Autodesk Inventor part; units mm, degrees
ref_plane "YZ Plane" through (0, 0, 0) normal (1, 0, 0) x (0, 1, 0)
ref_plane "XZ Plane" through (0, 0, 0) normal (0, 1, 0) x (-1, 0, 0)
ref_plane "XY Plane" through (0, 0, 0) normal (0, 0, 1) x (1, 0, 0)
sketch "Sketch1" plane through (0, 0, 0) normal (0, 1, 0) x (-1, 0, 0)
  circle A0 centre (368.3, 203.2) radius 2.54 construction
  circle A1 centre (368.3, 241.3) radius 3.302
  circle A2 centre (368.3, 127) radius 2.54 construction
  circle A3 centre (368.3, 88.9) radius 3.302
  circle A4 centre (368.3, 50.8) radius 2.54 construction
  circle A5 centre (368.3, 12.7) radius 3.302
  line L0 (190.5, 244.602) -> (330.2, 244.602)
  line L1 (330.2, 244.602) -> (190.5, 244.602)
  arc A6 (330.2, 237.998) -> (330.2, 244.602) centre (330.2, 241.3) ccw
  line L2 (190.5, 237.998) -> (330.2, 237.998)
  line L3 (381, 251.46) -> (381, 2.54)
  line L4 (378.46, 0) -> (355.6, 0)
  line L5 (355.6, 0) -> (355.6, 0)
  circle A7 centre (368.3, 38.1) radius 2.54 construction
  circle A8 centre (368.3, 63.5) radius 2.54 construction
  circle A9 centre (368.3, 127) radius 2.54 construction
  circle A10 centre (368.3, 114.3) radius 2.54 construction
  circle A11 centre (368.3, 139.7) radius 2.54 construction
  circle A12 centre (368.3, 203.2) radius 2.54 construction
  circle A13 centre (368.3, 190.5) radius 2.54 construction
  circle A14 centre (368.3, 215.9) radius 2.54 construction
  line L6 (355.6, 0) -> (355.6, 25.4) construction
  line L7 (355.6, 25.4) -> (381, 25.4) construction
  line L8 (368.3, 88.9) -> (355.6, 88.9) construction
  arc A15 (352.298, 76.2) -> (358.902, 76.2) centre (355.6, 76.2) ccw
  arc A16 (358.902, 101.6) -> (352.298, 101.6) centre (355.6, 101.6) ccw
  line L9 (358.902, 76.2) -> (358.902, 101.6)
  line L10 (352.298, 101.6) -> (352.298, 76.2)
  line L11 (368.3, 139.7) -> (368.3, 165.1) construction
  line L12 (368.3, 165.1) -> (355.6, 165.1) construction
  arc A17 (352.298, 152.4) -> (358.902, 152.4) centre (355.6, 152.4) ccw
  arc A18 (358.902, 177.8) -> (352.298, 177.8) centre (355.6, 177.8) ccw
  line L13 (358.902, 152.4) -> (358.902, 177.8)
  line L14 (352.298, 177.8) -> (352.298, 152.4)
  arc A19 (342.9, 12.7) -> (355.6, 0) centre (355.6, 12.7) ccw
  line L15 (378.46, 254) -> (190.5, 254)
  arc A20 (378.46, 0) -> (381, 2.54) centre (378.46, 2.54) ccw
  arc A21 (381, 251.46) -> (378.46, 254) centre (378.46, 251.46) ccw
  line L16 (190.5, 228.6) -> (190.5, 159.7209) construction
  line L17 (330.2, 215.9) -> (190.5, 215.9)
  line L18 (342.9, 12.7) -> (342.9, 203.2)
  arc A22 (342.9, 203.2) -> (330.2, 215.9) centre (330.2, 203.2) ccw
  circle A23 centre (12.7, 203.2) radius 2.54 construction
  circle A24 centre (12.7, 241.3) radius 3.302
  circle A25 centre (12.7, 127) radius 2.54 construction
  circle A26 centre (12.7, 88.9) radius 3.302
  circle A27 centre (12.7, 50.8) radius 2.54 construction
  circle A28 centre (12.7, 12.7) radius 3.302
  line L19 (190.5, 244.602) -> (50.8, 244.602)
  line L20 (50.8, 244.602) -> (190.5, 244.602)
  arc A29 (50.8, 244.602) -> (50.8, 237.998) centre (50.8, 241.3) ccw
  line L21 (190.5, 237.998) -> (50.8, 237.998)
  line L22 (0, 251.46) -> (0, 2.54)
  line L23 (2.54, 0) -> (25.4, 0)
  line L24 (25.4, 0) -> (25.4, 0)
  circle A30 centre (12.7, 38.1) radius 2.54 construction
  circle A31 centre (12.7, 63.5) radius 2.54 construction
  circle A32 centre (12.7, 139.7) radius 2.54 construction
  circle A33 centre (12.7, 127) radius 2.54 construction
  circle A34 centre (12.7, 114.3) radius 2.54 construction
  circle A35 centre (12.7, 215.9) radius 2.54 construction
  circle A36 centre (12.7, 203.2) radius 2.54 construction
  circle A37 centre (12.7, 190.5) radius 2.54 construction
  line L25 (25.4, 0) -> (25.4, 25.4) construction
  line L26 (25.4, 25.4) -> (0, 25.4) construction
  line L27 (12.7, 88.9) -> (25.4, 88.9) construction
  arc A38 (22.098, 76.2) -> (28.702, 76.2) centre (25.4, 76.2) ccw
  arc A39 (28.702, 101.6) -> (22.098, 101.6) centre (25.4, 101.6) ccw
  line L28 (22.098, 76.2) -> (22.098, 101.6)
  line L29 (28.702, 101.6) -> (28.702, 76.2)
  line L30 (12.7, 139.7) -> (12.7, 165.1) construction
  line L31 (12.7, 165.1) -> (25.4, 165.1) construction
  line L32 (22.098, 152.4) -> (22.098, 177.8)
  arc A40 (22.098, 152.4) -> (28.702, 152.4) centre (25.4, 152.4) ccw
  line L33 (28.702, 177.8) -> (28.702, 152.4)
  arc A41 (28.702, 177.8) -> (22.098, 177.8) centre (25.4, 177.8) ccw
  arc A42 (25.4, 0) -> (38.1, 12.7) centre (25.4, 12.7) ccw
  line L34 (2.54, 254) -> (190.5, 254)
  arc A43 (0, 2.54) -> (2.54, 0) centre (2.54, 2.54) ccw
  arc A44 (2.54, 254) -> (0, 251.46) centre (2.54, 251.46) ccw
  line L35 (50.8, 215.9) -> (190.5, 215.9)
  line L36 (38.1, 12.7) -> (38.1, 203.2)
  arc A45 (50.8, 215.9) -> (38.1, 203.2) centre (50.8, 203.2) ccw
  point P0 (381, 254)
  point P1 (381, 0)
  point P2 (342.9, 0)
  point P3 (342.9, 228.6)
  point P4 (0, 254)
  point P5 (0, 0)
  point P6 (38.1, 0)
  point P7 (38.1, 228.6)
  dimension "d2" = 12.7
  dimension "d3" = 228.6
  dimension "d6" = 25.4
  dimension "d7" = 25.4
  dimension "d8" = 12.7
  dimension "d10" = 25.4
  dimension "d12" = 12.7
  dimension "d17" = 12.7
ref_plane "Work Plane1" through (0, 6.35, 0) normal (0, 1, 0) x (1, 0, 0)
extrude "Extrusion4" add sketch "Sketch1" along normal blind 5.588
sketch "Sketch3" plane through (0, 5.588, 0) normal (0, 1, 0) x (1, 0, 0)
  arc A0 (-330.2, -237.998) -> (-330.2, -244.602) centre (-330.2, -241.3) ccw
  line L0 (-330.2, -237.998) -> (-50.8, -237.998)
  arc A1 (-50.8, -244.602) -> (-50.8, -237.998) centre (-50.8, -241.3) ccw
  line L1 (-50.8, -244.602) -> (-330.2, -244.602)
  line L2 (-22.098, -76.2) -> (-22.098, -101.6)
  arc A2 (-28.702, -101.6) -> (-22.098, -101.6) centre (-25.4, -101.6) ccw
  line L3 (-28.702, -101.6) -> (-28.702, -76.2)
  arc A3 (-22.098, -76.2) -> (-28.702, -76.2) centre (-25.4, -76.2) ccw
  line L4 (-28.702, -177.8) -> (-28.702, -152.4)
  arc A4 (-22.098, -152.4) -> (-28.702, -152.4) centre (-25.4, -152.4) ccw
  line L5 (-22.098, -152.4) -> (-22.098, -177.8)
  arc A5 (-28.702, -177.8) -> (-22.098, -177.8) centre (-25.4, -177.8) ccw
  line L6 (-352.298, -152.4) -> (-352.298, -177.8)
  arc A6 (-358.902, -177.8) -> (-352.298, -177.8) centre (-355.6, -177.8) ccw
  line L7 (-358.902, -177.8) -> (-358.902, -152.4)
  arc A7 (-352.298, -152.4) -> (-358.902, -152.4) centre (-355.6, -152.4) ccw
  line L8 (-358.902, -101.6) -> (-358.902, -76.2)
  arc A8 (-352.298, -76.2) -> (-358.902, -76.2) centre (-355.6, -76.2) ccw
  line L9 (-352.298, -76.2) -> (-352.298, -101.6)
  arc A9 (-358.902, -101.6) -> (-352.298, -101.6) centre (-355.6, -101.6) ccw
  circle A10 centre (-12.7, -88.9) radius 3.302
  circle A11 centre (-12.7, -12.7) radius 3.302
  circle A12 centre (-12.7, -241.3) radius 3.302
  circle A13 centre (-368.3, -12.7) radius 3.302
  circle A14 centre (-368.3, -88.9) radius 3.302
  circle A15 centre (-368.3, -241.3) radius 3.302
  line L10 (-355.6, 0) -> (-378.46, 0)
  arc A16 (-378.46, 0) -> (-381, -2.54) centre (-378.46, -2.54) ccw
  line L11 (-381, -2.54) -> (-381, -251.46)
  arc A17 (-381, -251.46) -> (-378.46, -254) centre (-378.46, -251.46) ccw
  line L12 (-378.46, -254) -> (-2.54, -254)
  arc A18 (-2.54, -254) -> (0, -251.46) centre (-2.54, -251.46) ccw
  line L13 (0, -251.46) -> (0, -2.54)
  arc A19 (0, -2.54) -> (-2.54, 0) centre (-2.54, -2.54) ccw
  line L14 (-2.54, 0) -> (-25.4, 0)
  arc A20 (-25.4, 0) -> (-38.1, -12.7) centre (-25.4, -12.7) ccw
  line L15 (-38.1, -12.7) -> (-38.1, -203.2)
  arc A21 (-50.8, -215.9) -> (-38.1, -203.2) centre (-50.8, -203.2) ccw
  line L16 (-50.8, -215.9) -> (-330.2, -215.9)
  arc A22 (-342.9, -203.2) -> (-330.2, -215.9) centre (-330.2, -203.2) ccw
  line L17 (-342.9, -203.2) -> (-342.9, -12.7)
  arc A23 (-342.9, -12.7) -> (-355.6, 0) centre (-355.6, -12.7) ccw
  circle A24 centre (-368.3, -12.7) radius 3.302
  line L18 (-368.3, -12.7) -> (-368.3, -38.1) construction
  line L19 (-368.3, -38.1) -> (-368.3, -50.8) construction
  line L20 (-368.3, -50.8) -> (-368.3, -63.5) construction
  line L21 (-368.3, -88.9) -> (-368.3, -114.3) construction
  line L22 (-368.3, -114.3) -> (-368.3, -127) construction
  line L23 (-368.3, -127) -> (-368.3, -139.7) construction
  line L24 (-368.3, -139.7) -> (-368.3, -165.1) construction
  line L25 (-368.3, -165.1) -> (-368.3, -190.5) construction
  line L26 (-368.3, -190.5) -> (-368.3, -203.2) construction
  line L27 (-368.3, -203.2) -> (-368.3, -215.9) construction
  line L28 (-368.3, -215.9) -> (-368.3, -241.3) construction
  line L29 (-12.7, -12.7) -> (-12.7, -38.1) construction
  line L30 (-12.7, -38.1) -> (-12.7, -50.8) construction
  line L31 (-12.7, -50.8) -> (-12.7, -63.5) construction
  line L32 (-12.7, -88.9) -> (-12.7, -114.3) construction
  line L33 (-12.7, -114.3) -> (-12.7, -127) construction
  line L34 (-12.7, -127) -> (-12.7, -139.7) construction
  line L35 (-12.7, -139.7) -> (-12.7, -165.1) construction
  line L36 (-12.7, -165.1) -> (-12.7, -190.5) construction
  line L37 (-12.7, -190.5) -> (-12.7, -203.2) construction
  line L38 (-12.7, -203.2) -> (-12.7, -215.9) construction
  line L39 (-12.7, -215.9) -> (-12.7, -241.3) construction
  point P0 (0, 0)
  dimension "d22" = 25.4
  dimension "d23" = 12.7
  dimension "d24" = 12.7
  dimension "d25" = 25.4
  dimension "d26" = 12.7
  dimension "d27" = 12.7
  dimension "d28" = 25.4
  dimension "d29" = 25.4
  dimension "d30" = 12.7
  dimension "d31" = 12.7
  dimension "d32" = 25.4
  dimension "d40" = 25.4
  dimension "d41" = 12.7
  dimension "d42" = 12.7
  dimension "d43" = 25.4
  dimension "d44" = 12.7
  dimension "d45" = 12.7
  dimension "d46" = 25.4
  dimension "d47" = 25.4
  dimension "d48" = 12.7
  dimension "d49" = 12.7
  dimension "d50" = 25.4
hole "Hole2" at (-368.3, 5.588, 38.1) at (-368.3, 5.588, 50.8) at (-368.3, 5.588, 63.5) at (-368.3, 5.588, 139.7) at (-368.3, 5.588, 127) at (-368.3, 5.588, 114.3) at (-368.3, 5.588, 215.9) at (-368.3, 5.588, 190.5) at (-368.3, 5.588, 203.2) at (-12.7, 5.588, 139.7) at (-12.7, 5.588, 215.9) at (-12.7, 5.588, 203.2) at (-12.7, 5.588, 190.5) at (-12.7, 5.588, 114.3) at (-12.7, 5.588, 127) at (-12.7, 5.588, 63.5) at (-12.7, 5.588, 50.8) at (-12.7, 5.588, 38.1) direction (0, -1, 0) diameter 4.9784 depth 13.97 tip angle 118
properties part number "vrRig_v08p1_base"
The model under review builds one solid part; all positions refer to its coordinate system, in mm. A direction names the side the tool comes from. Coordinates: 2 decimals unless noted, no trailing zeros. Order: outer loops, then holes, each group sorted by start corner. A loop starts at its lowest first (then second) coordinate and runs counter-clockwise, first axis right, second up. Notation, with made-up numbers: M -15.75,52 L 43.25,52 A18 cw 43.25,71 Z; hole C 55.25,38 d10. An arc over 180 degrees is marked long. One line per question, with ' | ' between items.
(1) Add section A-A, the plane x = -241.5. Write out the cut boundary in (y, z).
Geometry results:
outline: M 0,215.9 L 5.59,215.9 L 5.59,238 L 0,238 Z; M 0,244.6 L 5.59,244.6 L 5.59,254 L 0,254 Z
(2) For probe 1 along X at (y, z) = (3.6, 203); probe 2 along X at (y, z) = (1.55, 89); probe 3 along X at (y, z) = (2.2, 153), list the stretches that pass through material, from the lowest coordinate up. Write a range as from..to.
Geometry results:
probe 1: x = -381..-370.78, -365.82..-342.9, -38.1..-15.18, -10.22..0 | probe 2: x = -381..-371.6, -365..-358.9, -352.3..-342.9, -38.1..-28.7, -22.1..-16, -9.4..0 | probe 3: x = -381..-358.9, -352.3..-342.9, -38.1..-28.7, -22.1..0
(3) Insertion check: pin 1 (4.5 mm diameter, centred on x = -368.3, z = 203.2, fed in from +Y). The pin has a flat end and moves straight along its axis. Give the tip position at first contact, or say it passes through.
Geometry results:
pin 1: passes through
(4) Machinability: for faces 4 (the face through (-339.08, 2.75, 212.28)), 5 (the face through (-161, 0, 222)), which of the approach directions +Z, -Z, +X, -X, +Y, -Y give a long, thin tool a straight path to every point of the face, cutting with its end or side? Answer none if there is none.
Geometry results:
face 4: -Z, +Y, -Y | face 5: +Z, -Z, +X, -X, -Y
(5) The part is to be moulded in two halves that separate along X. For faces 1 (the face through (-346.72, 2.75, 3.62)), 2 (the face through (-41.72, 2.75, 212.08)), 3 (the face through (-161, 5.588, 222)), say which applies: +X half, -X half, draft (parallel to the pull), parting line (faces both ways), or undercut.
Geometry results:
face 1: undercut | face 2: undercut | face 3: draft
(6) Add section B-B, the plane y = 2. State how many separate pieces and enclosed holes the cut face has, then the cut area to 3 significant figures.
Geometry results:
separate pieces: 1 | enclosed holes: 29 | area: 27,700 mm²
